from build123d import *

# Parameters (mm, degrees)
BASPROSKE_W         = 7
BASPROSKE_H         = 13.5
TOOTHCUT_DEPTH      = 21.334699408
TEETHCUTS_COUNT     = 25
TEETHCUTS_ANGLE     = 345.6
BORSKE_R            = 0.4
BORE_DEPTH          = 50.0000508
SKETCH_1_R          = 5.1
CUT_EXTRUDE_1_DEPTH = 10
SKETCH_2_W          = 30
SKETCH_2_H          = 10
SKETCH_2_R          = 1.65
EXTRUDE_2_DEPTH     = 5
CUT_EXTRUDE_2_DEPTH = 2.5


with BuildPart() as part:
    # BasProSke → Base-Revolve (revolve)
    with BuildSketch(Plane(origin=(0, 0, 0), x_dir=(1, 0, 0), z_dir=(0, 1, 0)), mode=Mode.PRIVATE) as base_revolve_sk:
        with Locations((3.5, 6.75)):
            Rectangle(BASPROSKE_W, BASPROSKE_H)
    revolve(base_revolve_sk.sketch.rotate(Axis((-10, 0, 0), (1, 0, 0)), 180), axis=Axis((-10, 0, 0), (1, 0, 0)))

    # TooCutSke → ToothCut (cut, through all)
    with BuildSketch(Plane(origin=(0, 0, 0), x_dir=(0, 0, -1), z_dir=(1, 0, 0))):
        with BuildLine():
            ThreePointArc((0.480087995, 11.238750665), (0, 11.249), (-0.480087995, 11.238750665))
            ThreePointArc((-0.480087995, 11.238750665), (-0.821124963, 12.40220054), (-1.432168974, 13.449361962))
            ThreePointArc((-1.432168974, 13.449361962), (0, 13.5254), (1.432168974, 13.449361962))
            ThreePointArc((1.432168974, 13.449361962), (0.821124963, 12.40220054), (0.480087995, 11.238750665))
        make_face()
    toothcut = extrude(amount=TOOTHCUT_DEPTH, mode=Mode.SUBTRACT)

    # TeethCuts: ToothCut ×25 about axis
    teethcuts_axis = Axis((-10, 0, 0), (1, 0, 0))
    for i in range(1, TEETHCUTS_COUNT):
        add(toothcut.rotate(teethcuts_axis, i * TEETHCUTS_ANGLE / (TEETHCUTS_COUNT - 1)), mode=Mode.SUBTRACT)

    # BorSke → Bore (cut, symmetric)
    with BuildSketch(Plane(origin=(0, 0, 0), x_dir=(0, 0, -1), z_dir=(1, 0, 0))):
        with Locations(Location((0, 0, 0), (0, 0, 180))):
            Circle(BORSKE_R)
    extrude(amount=BORE_DEPTH, both=True, mode=Mode.SUBTRACT)

    # 草图1 → 切除-拉伸1 (cut)
    with BuildSketch(Plane(origin=(7, 0, 0), x_dir=(0, 0, -1), z_dir=(1, 0, 0))):
        Circle(SKETCH_1_R)
    extrude(amount=-CUT_EXTRUDE_1_DEPTH, mode=Mode.SUBTRACT)

    # 草图2 → 凸台-拉伸2 (add)
    with BuildSketch(Plane(origin=(7, 0, 0), x_dir=(0, 0, -1), z_dir=(1, 0, 0))):
        with Locations((-24, 0)):
            Rectangle(SKETCH_2_W, SKETCH_2_H)
        with Locations((-31, 0)):
            Circle(SKETCH_2_R, mode=Mode.SUBTRACT)
        with Locations((-19, 0)):
            Circle(SKETCH_2_R, mode=Mode.SUBTRACT)
    extrude(amount=-EXTRUDE_2_DEPTH)

    # 草图3 → 切除-拉伸2 (cut)
    with BuildSketch(Plane(origin=(7, 0, 0), x_dir=(0, 0, -1), z_dir=(1, 0, 0))):
        Polygon((-27.651368439, 0), (-29.325684219, 2.9), (-32.674315781, 2.9), (-34.348631561, 0), (-32.674315781, -2.9), (-29.325684219, -2.9), align=None)
        Polygon((-15.651368439, 0), (-17.325684219, 2.9), (-20.674315781, 2.9), (-22.348631561, 0), (-20.674315781, -2.9), (-17.325684219, -2.9), align=None)
    extrude(amount=-CUT_EXTRUDE_2_DEPTH, mode=Mode.SUBTRACT)


solid = part.part
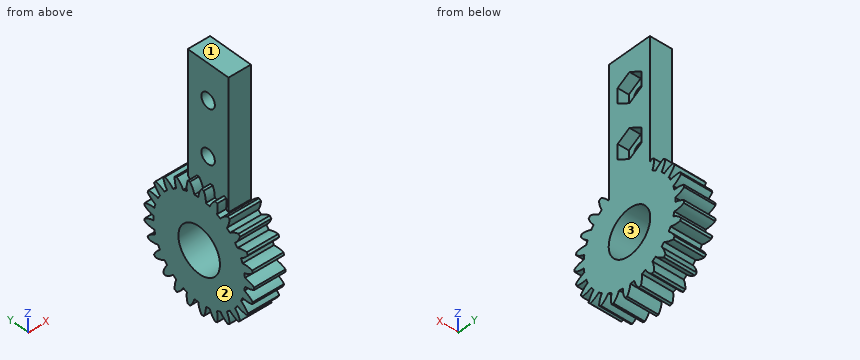
Part model, mm, in its own coordinate system. Face numbers are marked on the shaded views. Round coordinates to 2 decimals unless told otherwise and drop trailing zeros. Loops run counter-clockwise (first coordinate to the right, second up) from the corner with the lowest first, then second, coordinate; pieces in that order, holes last. Notation, with made-up numbers: (-34, 39) - (-8, 39) arc R22 cw to (-8, 77) - close; hole circle Ø1 at (75, 9). An arc over 180 degrees is marked (long way). Answer as a JSON object with one key per item and string values.
Item 1: Pin check, flat tips, straight feed: pin 1 (1.5 mm diameter, centred on x = 2.5, z = 21.5, fed in from +Y); pin 2 (3 mm diameter, centred on y = 2.5, z = 19.5, fed in from -X); pin 3 (4.5 mm diameter, centred on y = 0, z = 31, fed in from +X). Stop position of each tip, or through.
Output:
{"pin 1": "y = 5", "pin 2": "x = 2", "pin 3": "x = 4.5"}
Item 2: Band-saw the part on A-A on z = 31. List the corners of the cut face in (x, y), plus the area to 4 significant figures.
Output:
{"outline": "(2, -5) - (7, -5) - (7, -2.9) - (4.5, -2.9) - (4.5, -1.65) - (2, -1.65) - close; (2, 1.65) - (4.5, 1.65) - (4.5, 2.9) - (7, 2.9) - (7, 5) - (2, 5) - close", "area": "27.25 mm2"}
Item 3: Band-saw the part on C-C on x = 6.25. State how many separate pieces and enclosed holes the cut face has, plus the area to 3 significant figures.
Output:
{"separate pieces": "1", "enclosed holes": "3", "area": "608 mm2"}
Item 4: Pull direction Z, two halves, no side cores. Call the marked faces 1, 2 and 3: pulls with the +Z half, pulls with the -Z half, needs draft (parallel to the pull), parting line crosses it, or undercut.
Output:
{"face 1": "pulls with the +Z half", "face 2": "needs draft", "face 3": "undercut"}
Item 5: Wall check: L1, parallel to Z at x = 1, y = -9; L2, parallel to Y at x = 3.7, z = 31; L3, parallel to Z at x = 5, y = 9.75. Give the ranges that are in metal, low to high.
Output:
{"L1": "-9.24 to -7.2, -6.75 to 6.75, 7.2 to 9.24", "L2": "-5 to -1.65, 1.65 to 5", "L3": "-7.94 to -5.94, -5.61 to 5.61, 5.94 to 7.94"}
Item 6: Band-saw the part on B-B on y = 4.5. List the corners of the cut face in (x, z), plus the area to 3 significant figures.
Output:
{"outline": "(0, -11.41) - (7, -11.41) - (7, -2.4) - (0, -2.4) - close; (0, 2.4) - (7, 2.4) - (7, 39) - (2, 39) - (2, 11.41) - (0, 11.41) - close", "area": "264 mm2"}
